from build123d import *


# Not quite as in the source:
# - a fillet or chamfer that OpenCascade refuses, or shapes differently, is made with other operations: its cross-section is extruded or revolved along the edge and cut away or added


with BuildPart() as f2:
    # F0 (on Front) → F2 (revolve)
    with BuildSketch(Plane.XZ):
        with BuildLine():
            Line((-30.0974734128, 0), (8.0025265872, 0))
            Line((8.0025265872, 0), (8.0025265872, 76.2))
            Line((8.0025265872, 76.2), (-30.0974734128, 76.2))
            Line((-30.0974734128, 76.2), (-30.0974734128, 71.8881083488))
            ThreePointArc((-30.0974734128, 71.8881083488), (-23.7474734128, 65.5381083488), (-30.0974734128, 59.1881083488))
            Line((-30.0974734128, 59.1881083488), (-30.0974734128, 15.4437847272))
            ThreePointArc((-30.0974734128, 15.4437847272), (-23.7474734128, 9.0937847272), (-30.0974734128, 2.7437847272))
            Line((-30.0974734128, 2.7437847272), (-30.0974734128, 0))
        make_face()
    revolve(axis=Axis((8.0025265872, 0, 38.1), (0, 0, 1)))

    # F3: chamfer of 5.08 on 2 edges, made by hand

    # F3_s1 → F3_t2 (revolve, cut)
    with BuildSketch(Plane.XZ):
        Polygon((-25.0174734128, 76.2), (-30.0974734128, 71.12), (-30.0974734128, 76.2), align=None)
    revolve(axis=Axis((8.0025265872, 0, 76.2), (0, 0, 1)), mode=Mode.SUBTRACT)

    # F3_s3 → F3_t4 (revolve, cut)
    with BuildSketch(Plane.XZ):
        Polygon((-30.0974734128, 5.08), (-25.0174734128, 0), (-30.0974734128, 0), align=None)
    revolve(axis=Axis((8.0025265872, 0, 0), (0, 0, 1)), mode=Mode.SUBTRACT)


solid = f2.part
Build history of the part. All positions in model axes, mm. Coordinates: 2 decimals unless noted, no trailing zeros. Write each loop counter-clockwise with the first axis right and the second up, starting at its lowest first coordinate (ties: lowest second). Pieces come first, ordered by that corner, then holes.
(1) Cut at B-B on z = 36.5. List the corners of the cut face in (x, y).
(2) Cut at A-A on y = 0. List the corners of the cut face in (x, z).
(3) Cut at C-C on z = 5. List the corners of the cut face in (x, y), and give its area (3 significant figures).
(4) Pin check, flat tips, straight feed: pin 1 Ø12 at (y, z) = (17, 29.5) entering from +X; pin 2 Ø12 at (x, z) = (27, 43) entering from +Y; pin 3 Ø1.5 at (x, y) = (-22, 19.5) entering from +Z. Stop position of each tip, or through.
(5) Drill centre lines: line 1 (Z direction, x = 15.5, y = 32); line 2 (Y direction, x = 27, z = 52); line 3 (Z direction, x = 36.5, y = -18.5). Where is each one in solid material? Low to high.
Working result:
1. outline: circle Ø76.2 at (8, 0)
2. outline: (-30.1, 15.44) arc R6.35 cw to (-28.09, 3.07) - (-25.02, 0) - (41.02, 0) - (44.09, 3.07) arc R6.35 cw to (46.1, 15.44) - (46.1, 59.19) arc R6.35 cw to (45.38, 71.85) - (41.02, 76.2) - (-25.02, 76.2) - (-29.37, 71.85) arc R6.35 cw to (-30.1, 59.19) - close
3. outline: circle Ø66.49 at (8, 0)
3. area: 3,470 mm2
4. pin 1: stops at x = 44.48
4. pin 2: stops at y = 35.81
4. pin 3: stops at z = 74.19
5. line 1: z = 0 to 5.5, 12.69 to 61.94, 69.13 to 76.2
5. line 2: y = -33.03 to 33.03
5. line 3: z = 0.96 to 4.27, 13.92 to 60.71, 70.37 to 75.24
